Job drawing, mm, ordinate dimensions from the low corner. One solid piece. A direction names the side the tool comes from. Give positions to 0.01 mm unless a question says otherwise; leave off trailing zeros. Write each loop counter-clockwise with the first axis right and the second up, starting at its lowest first coordinate (ties: lowest second). Pieces come first, ordered by that corner, then holes. Notation, with made-up numbers: M 76.5,25.5 L 126.5,25.5 A29 cw 126.5,50.5 Z; hole C 68,81 d1. An arc over 180 degrees is marked long. Use a Markdown table: item, result.
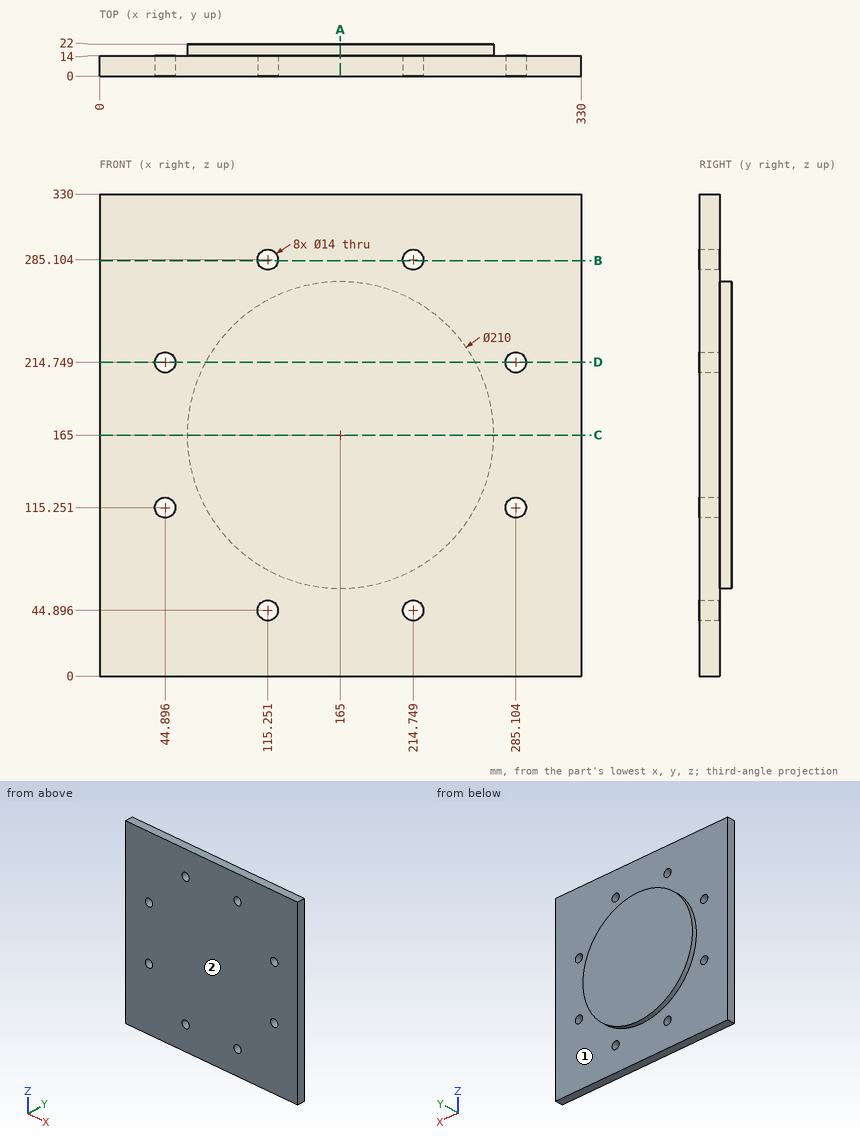
1. Cut at A-A, the plane x = 165. Give the cut face in (y, z), then the cut area to 3 significant figures.
Findings below:
| item | result |
|---|---|
| outline | M 0,0 L 14,0 L 14,60 L 22,60 L 22,270 L 14,270 L 14,330 L 0,330 Z |
| area | 6,300 mm2 |
2. Tool access for the marked faces 1 and 2: list every direction of +Z, -Z, +X, -X, +Y, -Y with a clear straight run to the whole face (end or side of a thin tool).
Findings below:
| item | result |
|---|---|
| face 1 | +Y |
| face 2 | +Z, -Z, +X, -X, -Y |
3. Cut at B-B, the plane z = 284.5. Give the cut face in (x, y) (1 decimal).
Findings below:
| item | result |
|---|---|
| outline | M 0,0 L 108.3,0 L 108.3,14 L 0,14 Z; M 122.2,0 L 207.8,0 L 207.8,14 L 122.2,14 Z; M 221.7,0 L 330,0 L 330,14 L 221.7,14 Z |
4. Cut at C-C, the plane z = 165. Give the cut face in (x, y).
Findings below:
| item | result |
|---|---|
| outline | M 0,0 L 330,0 L 330,14 L 270,14 L 270,22 L 60,22 L 60,14 L 0,14 Z |
5. Cut at D-D, the plane z = 215. Give the cut face in (x, y), then the cut area to 3 significant figures.
Findings below:
| item | result |
|---|---|
| outline | M 0,0 L 37.9,0 L 37.9,14 L 0,14 Z; M 51.89,0 L 278.11,0 L 278.11,14 L 257.33,14 L 257.33,22 L 72.67,22 L 72.67,14 L 51.89,14 Z; M 292.1,0 L 330,0 L 330,14 L 292.1,14 Z |
| area | 5,710 mm2 |
6. Drill centre lines: L1, parallel to Y at x = 25, z = 190.5; L2, parallel to Z at x = 239, y = 20.5; L3, parallel to Z at x = 108, y = 18.25. Where is each one in solid material? Low to high.
Findings below:
| item | result |
|---|---|
| L1 | 0 to 14 |
| L2 | 90.51 to 239.49 |
| L3 | 76.82 to 253.18 |
7. Drop flat-ended pins along their axis: P1, Ø1, axis at y = 12, z = 103, coming from the -X side; P2, Ø1, axis at x = 164, y = 16.5, coming from the +Z side; P3, Ø8.5, axis at x = 285.1, z = 115.25, coming from the +Y side; P4, Ø16, axis at x = 115.25, z = 44.9, coming from the +Y side. Give the stop position or say it passes through.
Findings below:
| item | result |
|---|---|
| P1 | x = 0 |
| P2 | z = 270 |
| P3 | through |
| P4 | y = 14 |
